Answer from the drawing. Dimensions are ordinates in mm from the lowest x, y and z of the part. A direction names the side the tool comes from. Coordinates: 2 decimals unless noted, no trailing zeros. Write each loop counter-clockwise with the first axis right and the second up, starting at its lowest first coordinate (ties: lowest second). Pieces come first, ordered by that corner, then holes.
1) Each of these flat-tipped pins is pushed along its axis until it touches: pin 1 Ø6 at (x, z) = (31, 16) entering from -Y; pin 2 Ø4 at (x, z) = (36, 36.5) entering from -Y. Where does it stop, or does it pass through?
2) Which of the six approach directions +Z, -Z, +X, -X, +Y, -Y give full straight-line access (tool end or side, diameter ignored) to the marked faces 1 and 2?
3) Determine the mould class of the marked faces 3, 4 and 5 for opening direction Z: +Z half, -Z half, draft (parallel to the pull), parting line (faces both ways), or undercut.
4) The part is cut by section B-B (y = 31.5). Determine the outline of the cut face in (x, z).
5) The part is cut by section A-A (x = 30). Determine the outline of the cut face in (y, z).
6) The part is cut by section C-C (z = 20). Determine the outline of the cut face in (x, y), then the cut area to 3 significant figures.
7) Find the intervals of material crossed by line 1 (Z direction, x = 28.5, y = 11.5); line 2 (X direction, y = 24, z = 38); line 3 (Z direction, x = 60, y = 26), in increasing order.
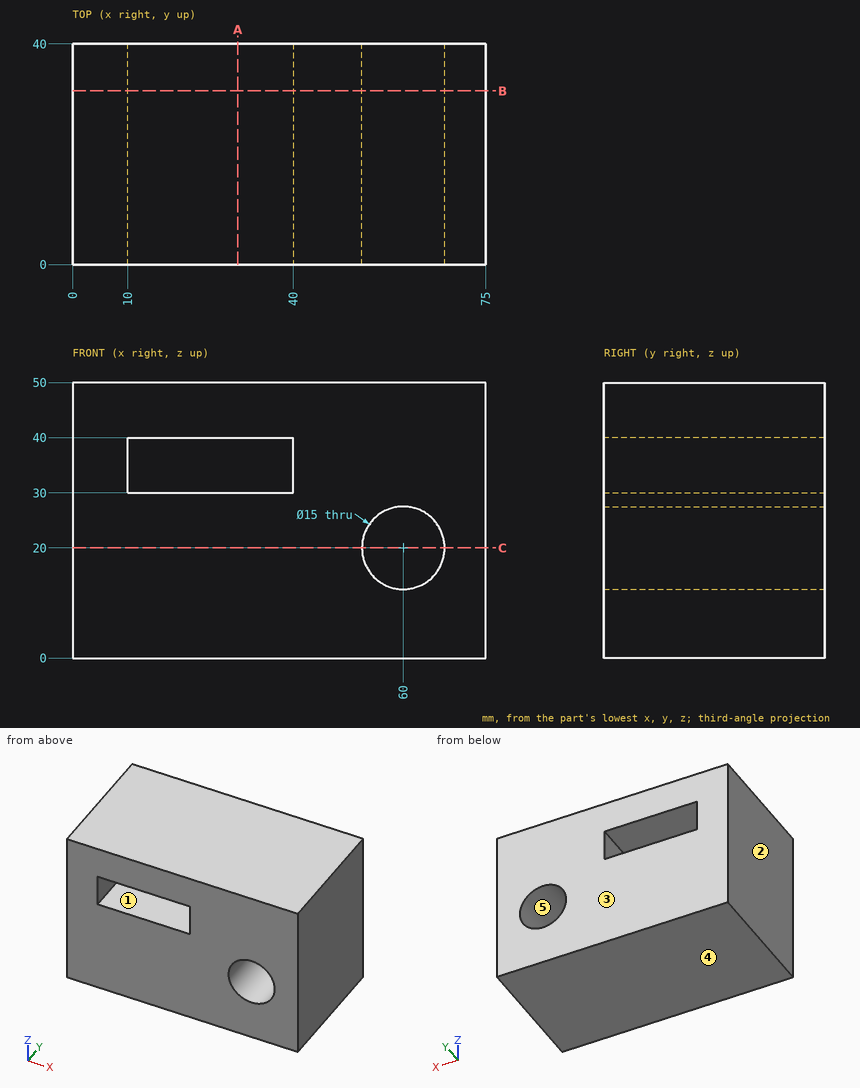
Reported:
1. pin 1: stops at y = 0
1. pin 2: passes through
2. face 1: +Y, -Y
2. face 2: +Z, -Z, -X, +Y, -Y
3. face 3: draft
3. face 4: -Z half
3. face 5: undercut
4. outline: (0, 0) - (75, 0) - (75, 50) - (0, 50) - close; hole (10, 30) - (40, 30) - (40, 40) - (10, 40) - close; hole circle Ø15 at (60, 20)
5. outline: (0, 0) - (40, 0) - (40, 30) - (0, 30) - close; (0, 40) - (40, 40) - (40, 50) - (0, 50) - close
6. outline: (0, 0) - (52.5, 0) - (52.5, 40) - (0, 40) - close; (67.5, 0) - (75, 0) - (75, 40) - (67.5, 40) - close
6. area: 2,400 mm2
7. line 1: z = 0 to 30, 40 to 50
7. line 2: x = 0 to 10, 40 to 75
7. line 3: z = 0 to 12.5, 27.5 to 50
